Source: CAD feature listing. Evaluate the final solid. Frame: model axes, mm. Face numbers are marked on the shaded views. A direction names the side the tool comes from. Coordinates: 2 decimals unless noted, no trailing zeros. Write each loop counter-clockwise with the first axis right and the second up, starting at its lowest first coordinate (ties: lowest second). Pieces come first, ordered by that corner, then holes. Notation, with made-up numbers: (27.5, -23) - (81.5, -23) arc R20 ccw to (81.5, -1) - close; hole circle Ø7 at (17.25, -19.75). An arc over 180 degrees is marked (long way). One line per item, written item: value.
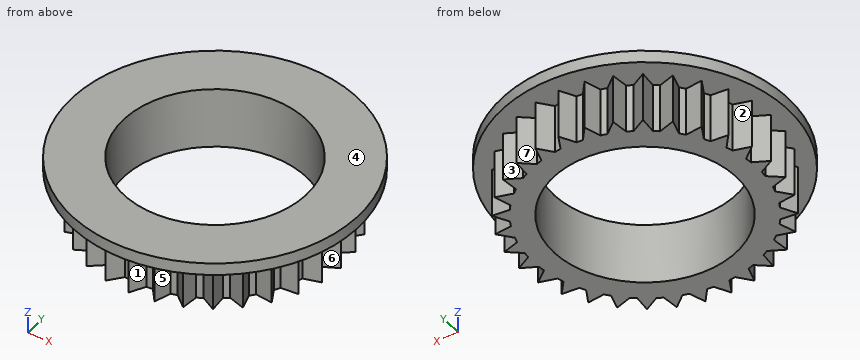
from build123d import *

# Parameters (mm, degrees)
BOSS_EXTRUDE1_DEPTH = 8
SKETCH3_R           = 23.5
BOSS_EXTRUDE2_DEPTH = 2
SKETCH5_R           = 15
CUT_EXTRUDE2_DEPTH  = 12


with BuildPart() as part:
    # Sketch1 → Boss-Extrude1 (new body)
    with BuildSketch(Plane.XY):
        with BuildLine():
            Line((0, 20.911393532), (1.305419533, 18.453885223))
            ThreePointArc((1.305419533, 18.453885223), (1.813317096, 18.410917443), (2.319838147, 18.353973711))
            Line((2.319838147, 18.353973711), (4.079610498, 20.509586969))
            Line((4.079610498, 20.509586969), (4.880510674, 17.844624276))
            ThreePointArc((4.880510674, 17.844624276), (5.370266529, 17.703396211), (5.855945749, 17.548729281))
            Line((5.855945749, 17.548729281), (8.002443852, 19.319608481))
            Line((8.002443852, 19.319608481), (8.268046526, 16.549604426))
            ThreePointArc((8.268046526, 16.549604426), (8.720839631, 16.31554339), (9.16701264, 16.069097027))
            Line((9.16701264, 16.069097027), (11.617747778, 17.387188273))
            Line((11.617747778, 17.387188273), (11.337845987, 14.618592558))
            ThreePointArc((11.337845987, 14.618592558), (11.736275757, 14.300693387), (12.125796376, 13.971938385))
            Line((12.125796376, 13.971938385), (14.786588171, 14.786588171))
            Line((14.786588171, 14.786588171), (13.971938385, 12.125796376))
            ThreePointArc((13.971938385, 12.125796376), (14.300693387, 11.736275757), (14.618592558, 11.337845987))
            Line((14.618592558, 11.337845987), (17.387188273, 11.617747778))
            Line((17.387188273, 11.617747778), (16.069097027, 9.16701264))
            ThreePointArc((16.069097027, 9.16701264), (16.31554339, 8.720839631), (16.549604426, 8.268046526))
            Line((16.549604426, 8.268046526), (19.319608481, 8.002443852))
            Line((19.319608481, 8.002443852), (17.548729281, 5.855945749))
            ThreePointArc((17.548729281, 5.855945749), (17.703396211, 5.370266529), (17.844624276, 4.880510674))
            Line((17.844624276, 4.880510674), (20.509586969, 4.079610498))
            Line((20.509586969, 4.079610498), (18.353973711, 2.319838147))
            ThreePointArc((18.353973711, 2.319838147), (18.410917443, 1.813317096), (18.453885223, 1.305419533))
            Line((18.453885223, 1.305419533), (20.911393532, 0))
            Line((20.911393532, 0), (18.453885223, -1.305419533))
            ThreePointArc((18.453885223, -1.305419533), (18.410917443, -1.813317096), (18.353973711, -2.319838147))
            Line((18.353973711, -2.319838147), (20.509586969, -4.079610498))
            Line((20.509586969, -4.079610498), (17.844624276, -4.880510674))
            ThreePointArc((17.844624276, -4.880510674), (17.703396211, -5.370266529), (17.548729281, -5.855945749))
            Line((17.548729281, -5.855945749), (19.319608481, -8.002443852))
            Line((19.319608481, -8.002443852), (16.549604426, -8.268046526))
            ThreePointArc((16.549604426, -8.268046526), (16.31554339, -8.720839631), (16.069097027, -9.16701264))
            Line((16.069097027, -9.16701264), (17.387188273, -11.617747778))
            Line((17.387188273, -11.617747778), (14.618592558, -11.337845987))
            ThreePointArc((14.618592558, -11.337845987), (14.300693387, -11.736275757), (13.971938385, -12.125796376))
            Line((13.971938385, -12.125796376), (14.786588171, -14.786588171))
            Line((14.786588171, -14.786588171), (12.125796376, -13.971938385))
            ThreePointArc((12.125796376, -13.971938385), (11.736275757, -14.300693387), (11.337845987, -14.618592558))
            Line((11.337845987, -14.618592558), (11.617747778, -17.387188273))
            Line((11.617747778, -17.387188273), (9.16701264, -16.069097027))
            ThreePointArc((9.16701264, -16.069097027), (8.720839631, -16.31554339), (8.268046526, -16.549604426))
            Line((8.268046526, -16.549604426), (8.002443852, -19.319608481))
            Line((8.002443852, -19.319608481), (5.855945749, -17.548729281))
            ThreePointArc((5.855945749, -17.548729281), (5.370266529, -17.703396211), (4.880510674, -17.844624276))
            Line((4.880510674, -17.844624276), (4.079610498, -20.509586969))
            Line((4.079610498, -20.509586969), (2.319838147, -18.353973711))
            ThreePointArc((2.319838147, -18.353973711), (1.813317096, -18.410917443), (1.305419533, -18.453885223))
            Line((1.305419533, -18.453885223), (0, -20.911393532))
            Line((0, -20.911393532), (-1.305419533, -18.453885223))
            ThreePointArc((-1.305419533, -18.453885223), (-1.813317096, -18.410917443), (-2.319838147, -18.353973711))
            Line((-2.319838147, -18.353973711), (-4.079610498, -20.509586969))
            Line((-4.079610498, -20.509586969), (-4.880510674, -17.844624276))
            ThreePointArc((-4.880510674, -17.844624276), (-5.370266529, -17.703396211), (-5.855945749, -17.548729281))
            Line((-5.855945749, -17.548729281), (-8.002443852, -19.319608481))
            Line((-8.002443852, -19.319608481), (-8.268046526, -16.549604426))
            ThreePointArc((-8.268046526, -16.549604426), (-8.720839631, -16.31554339), (-9.16701264, -16.069097027))
            Line((-9.16701264, -16.069097027), (-11.617747778, -17.387188273))
            Line((-11.617747778, -17.387188273), (-11.337845987, -14.618592558))
            ThreePointArc((-11.337845987, -14.618592558), (-11.736275757, -14.300693387), (-12.125796376, -13.971938385))
            Line((-12.125796376, -13.971938385), (-14.786588171, -14.786588171))
            Line((-14.786588171, -14.786588171), (-13.971938385, -12.125796376))
            ThreePointArc((-13.971938385, -12.125796376), (-14.300693387, -11.736275757), (-14.618592558, -11.337845987))
            Line((-14.618592558, -11.337845987), (-17.387188273, -11.617747778))
            Line((-17.387188273, -11.617747778), (-16.069097027, -9.16701264))
            ThreePointArc((-16.069097027, -9.16701264), (-16.31554339, -8.720839631), (-16.549604426, -8.268046526))
            Line((-16.549604426, -8.268046526), (-19.319608481, -8.002443852))
            Line((-19.319608481, -8.002443852), (-17.548729281, -5.855945749))
            ThreePointArc((-17.548729281, -5.855945749), (-17.703396211, -5.370266529), (-17.844624276, -4.880510674))
            Line((-17.844624276, -4.880510674), (-20.509586969, -4.079610498))
            Line((-20.509586969, -4.079610498), (-18.353973711, -2.319838147))
            ThreePointArc((-18.353973711, -2.319838147), (-18.410917443, -1.813317096), (-18.453885223, -1.305419533))
            Line((-18.453885223, -1.305419533), (-20.911393532, 0))
            Line((-20.911393532, 0), (-18.453885223, 1.305419533))
            ThreePointArc((-18.453885223, 1.305419533), (-18.410917443, 1.813317096), (-18.353973711, 2.319838147))
            Line((-18.353973711, 2.319838147), (-20.509586969, 4.079610498))
            Line((-20.509586969, 4.079610498), (-17.844624276, 4.880510674))
            ThreePointArc((-17.844624276, 4.880510674), (-17.703396211, 5.370266529), (-17.548729281, 5.855945749))
            Line((-17.548729281, 5.855945749), (-19.319608481, 8.002443852))
            Line((-19.319608481, 8.002443852), (-16.549604426, 8.268046526))
            ThreePointArc((-16.549604426, 8.268046526), (-16.31554339, 8.720839631), (-16.069097027, 9.16701264))
            Line((-16.069097027, 9.16701264), (-17.387188273, 11.617747778))
            Line((-17.387188273, 11.617747778), (-14.618592558, 11.337845987))
            ThreePointArc((-14.618592558, 11.337845987), (-14.300693387, 11.736275757), (-13.971938385, 12.125796376))
            Line((-13.971938385, 12.125796376), (-14.786588171, 14.786588171))
            Line((-14.786588171, 14.786588171), (-12.125796376, 13.971938385))
            ThreePointArc((-12.125796376, 13.971938385), (-11.736275757, 14.300693387), (-11.337845987, 14.618592558))
            Line((-11.337845987, 14.618592558), (-11.617747778, 17.387188273))
            Line((-11.617747778, 17.387188273), (-9.16701264, 16.069097027))
            ThreePointArc((-9.16701264, 16.069097027), (-8.720839631, 16.31554339), (-8.268046526, 16.549604426))
            Line((-8.268046526, 16.549604426), (-8.002443852, 19.319608481))
            Line((-8.002443852, 19.319608481), (-5.855945749, 17.548729281))
            ThreePointArc((-5.855945749, 17.548729281), (-5.370266529, 17.703396211), (-4.880510674, 17.844624276))
            Line((-4.880510674, 17.844624276), (-4.079610498, 20.509586969))
            Line((-4.079610498, 20.509586969), (-2.319838147, 18.353973711))
            ThreePointArc((-2.319838147, 18.353973711), (-1.813317096, 18.410917443), (-1.305419533, 18.453885223))
            Line((-1.305419533, 18.453885223), (0, 20.911393532))
        make_face()
    extrude(amount=BOSS_EXTRUDE1_DEPTH)

    # Sketch3 → Boss-Extrude2 (add)
    with BuildSketch(Plane.XY.offset(8)):
        Circle(SKETCH3_R)
    extrude(amount=BOSS_EXTRUDE2_DEPTH)

    # Sketch5 → Cut-Extrude2 (cut)
    with BuildSketch(Plane.XY.offset(10)):
        Circle(SKETCH5_R)
    extrude(amount=-CUT_EXTRUDE2_DEPTH, mode=Mode.SUBTRACT)


solid = part.part
1) Draft query along Y for the marked faces 4, 5, 6 and 7. Return one class per face: released by +Y, released by -Y, zero draft, split by the parting line, or undercut.
Values found:
face 4: zero draft
face 5: released by -Y
face 6: undercut
face 7: released by +Y
2) Section query A-A on y = 10.5. Output: boundary loops of the cut face in (x, z).
Values found:
outline: (-21.02, 8) - (-16.79, 8) - (-16.79, 0) - (-10.71, 0) - (-10.71, 10) - (-21.02, 10) - close; (10.71, 0) - (16.79, 0) - (16.79, 8) - (21.02, 8) - (21.02, 10) - (10.71, 10) - close
3) Section query B-B on z = 9. Output: boundary loops of the cut face in (x, y), then the cut area to 3 significant figures.
Values found:
outline: circle Ø47 at (0, 0); hole circle Ø30 at (0, 0)
area: 1,030 mm2
4) Reachability of the marked faces 1, 2 and 3 from +Z, -Z, +X, -X, +Y, -Y: full face, straight path, thin tool, end or side. Return the list, or none.
Values found:
face 1: -Z, -Y
face 2: -Z, -X
face 3: -Z, +Y
5) Contact query for flat-ended pins moving along their axis: P1, Ø4, axis at x = 9.5, z = 1, coming from the +Y side; P2, Ø6, axis at x = 5, z = 2.5, coming from the -Y side; P3, Ø2, axis at x = -2, z = 2.5, coming from the +Y side. Output: stop coordinate, or through.
Values found:
P1: y = 19.32
P2: y = -20.51
P3: y = 19.19
6) Material intervals for line 1 (Y direction, x = 18.5, z = 3); line 2 (Z direction, x = 18.5, y = 11.5); line 3 (Y direction, x = 7, z = 9), sorted ascending.
Values found:
line 1: -8.08 to -7.01, -4.68 to -2.44, -1.28 to 1.28, 2.44 to 4.68, 7.01 to 8.08
line 2: 8 to 10
line 3: -22.43 to -13.27, 13.27 to 22.43
7) Section query C-C on y = -6.5. Output: boundary loops of the cut face in (x, z).
Values found:
outline: (-22.58, 8) - (-18.08, 8) - (-18.08, 0) - (-13.52, 0) - (-13.52, 10) - (-22.58, 10) - close; (13.52, 0) - (18.08, 0) - (18.08, 8) - (22.58, 8) - (22.58, 10) - (13.52, 10) - close
